from build123d import *

# Parameters (mm, degrees)
F0_R     = 17.5
F1_DEPTH = 45
F1_TAPER = -5
F3_R     = 6
F4_DEPTH = 35
F4_TAPER = 1
F5_SIZE  = 5


with BuildPart() as f1:
    # F0 (on Top) → F1 (new body)
    with BuildSketch(Plane.XY):
        Circle(F0_R)
    extrude(amount=F1_DEPTH, taper=F1_TAPER)

    # F3 (on face) → F4 (cut)
    with BuildSketch(Plane.XY.offset(45)):
        Circle(F3_R)
    extrude(amount=-F4_DEPTH, taper=F4_TAPER, mode=Mode.SUBTRACT)

    # F5
    f5_edges = [f1.edges().sort_by_distance(p)[0] for p in [
        (-5.389073, 0, 10),
    ]]
    chamfer(f5_edges, length=F5_SIZE)

    # F2 (on Front) → F6 (revolve, cut)
    with BuildSketch(Plane.XZ):
        with BuildLine():
            Line((0, 34.8251537271), (0, 64.8251537271))
            add(Edge.make_bspline(
                [(0, 64.8251537271), (-20, 64.8251537271), (-20, 49.8251537271), (-20, 34.8251537271), (0, 34.8251537271)],
                knots=[1.5707963268, 1.5707963268, 1.5707963268, 3.1415926536, 3.1415926536, 4.7123889804, 4.7123889804, 4.7123889804], degree=2, weights=[1, 0.7071067812, 1, 0.7071067812, 1]))
        make_face()
    revolve(axis=Axis((0, 0, 39.5477935672), (0, 0, 1)), mode=Mode.SUBTRACT)


solid = f1.part
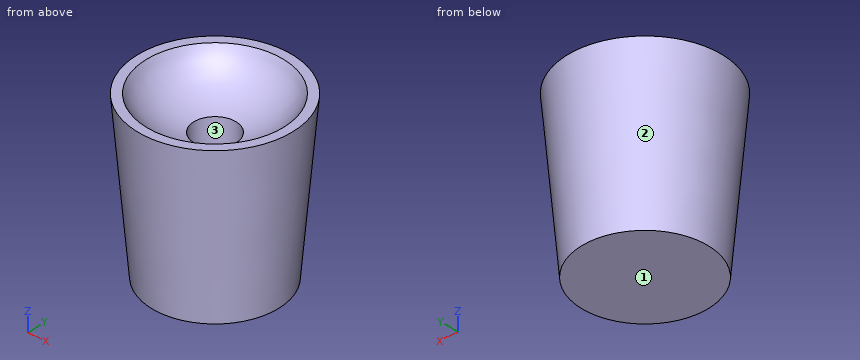
Here's how the part is built. I have some questions about the finished solid (model axes, mm). Face numbers are marked on the shaded views. Give positions to 0.01 mm unless a question says otherwise; leave off trailing zeros. Order: outer loops, then holes, each group sorted by start corner. A loop starts at its lowest first (then second) coordinate and runs counter-clockwise, first axis right, second up. Notation, with made-up numbers: (81, 53.5) -> (91, 53.5) arc R14 cw to (91, 63.5) -> close; hole circle Ø7 at (-0.5, 81.25). An arc over 180 degrees is marked (long way). Use a Markdown table: item, result. Add a question column.
Item 1: If we mould it in two halves opening along X, with no side actions, what happens to the marked faces 1, 2 and 3? For each: pulls with the +X half, pulls with the -X half, needs draft (parallel to the pull), parting line crosses it, or undercut.
Item 2: Imagine slicing it at A-A on z = 23.5. Please give me the cut outline in (x, y), plus the area to 3 significant figures.
Item 3: Will these pins go through, and if not, where does the flat tip stop? pin 1 (4 mm diameter, centred on x = -10.5, z = 33, fed in from -Y); pin 2 (5 mm diameter, centred on x = -8.5, y = -12, fed in from +Z); pin 3 (8 mm diameter, centred on y = 17, z = 7.5, fed in from +X).
Item 4: Imagine slicing it at B-B on z = 33.5. Please give me the cut outline in (x, y).
Item 5: I need wall thicknesses on line 1 (X direction, y = 6.5, z = 40.5); line 2 (Y direction, x = -1, z = 35); line 3 (Y direction, x = 2.5, z = 42.5). Which ranges of each line are inside material? Lowest first, please.
Data:
| question | item | result |
|---|---|---|
| 1 | face 1 | needs draft |
| 1 | face 2 | parting line crosses it |
| 1 | face 3 | undercut |
| 2 | outline | circle Ø39.11 at (0, 0); hole circle Ø11.25 at (0, 0) |
| 2 | area | 1,100 mm² |
| 3 | pin 1 | stops at y = -18.55 |
| 3 | pin 2 | stops at z = 42.18 |
| 3 | pin 3 | stops at x = 12.71 |
| 4 | outline | circle Ø40.86 at (0, 0); hole circle Ø11.6 at (0, 0) |
| 5 | line 1 | x = -20.01 to -14.25, 14.25 to 20.01 |
| 5 | line 2 | y = -20.54 to -5.74, 5.74 to 20.54 |
| 5 | line 3 | y = -21.07 to -17.27, 17.27 to 21.07 |
